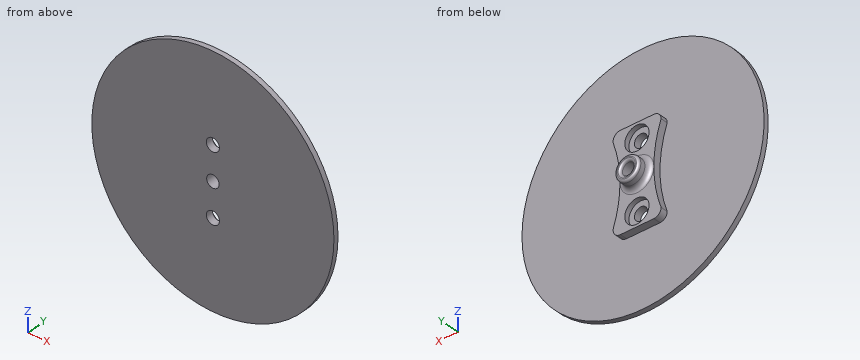
Autodesk Inventor part; units mm, degrees
ref_plane "YZ Plane" through (0, 0, 0) normal (1, 0, 0) x (0, 1, 0)
ref_plane "XZ Plane" through (0, 0, 0) normal (0, 1, 0) x (-1, 0, 0)
ref_plane "XY Plane" through (0, 0, 0) normal (0, 0, 1) x (1, 0, 0)
sketch "Boceto1" plane through (0, 0, 0) normal (0, 1, 0) x (-1, 0, 0)
  circle A0 centre (0, 0) radius 2.7
  line L0 (10, 20) -> (-10, 20)
  line L1 (-10, 20) -> (-10, -20)
  line L2 (-10, -20) -> (10, -20)
  line L3 (10, -20) -> (10, 20)
  line L4 (10, 20) -> (-10, -20) construction
  line L5 (-10, 20) -> (10, -20) construction
  circle A1 centre (0, 14) radius 2.7
  circle A2 centre (0, -14) radius 2.7
  dimension "d0" = 5.4
  dimension "d1" = 20
  dimension "d2" = 40
  dimension "d3" = 6
  dimension "d4" = 6
extrude "Extrusión1" add sketch "Boceto1" along normal blind 5
sketch "Boceto2" plane through (0, 5, 0) normal (0, 1, 0) x (1, 0, 0)
  circle A0 centre (0, 0) radius 2.7
  circle A1 centre (0, 0) radius 2.7
  circle A2 centre (0, 0) radius 5
  dimension "d21" = 2
  dimension "d22" = 0
  dimension "d7" = 10
extrude "Extrusión2" add sketch "Boceto2" along normal blind 5
sketch "Boceto3" plane through (0, 10, 0) normal (0, 1, 0) x (1, 0, 0)
  circle A0 centre (0, 0) radius 2.575
  circle A1 centre (0, 0) radius 2.7
  dimension "d10" = 5.15
extrude "Extrusión3" add sketch "Boceto3" against normal up to surface (10 mm away)
fillet "Empalme1" radius 3 4 edges at (-10, 2.5, -20) (10, 2.5, -20) (10, 2.5, 20) (-10, 2.5, 20)
fillet "Empalme2" radius 2 1 edges at (-5, 5, 0)
sketch "Boceto4" plane through (0, 5, 0) normal (0, 1, 0) x (1, 0, 0)
  line L0 (10, -17) -> (10, 17)
  arc A0 (10, 17) -> (10, -17) centre (56.6667, 0) ccw
  line L1 (10, -17) -> (10, 17)
  line L2 (-10, 17) -> (-10, -17)
  arc A1 (-7, 20) -> (-10, 17) centre (-7, 17) ccw
  arc A2 (-10, -17) -> (-10, 17) centre (-56.6667, 0) ccw
  line L3 (-10, 17) -> (-10, -17)
  point P0 (0, 0)
extrude "Extrusión4" cut sketch "Boceto4" against normal through all
fillet "Empalme3" radius 3 2 edges at (10, 2.5, 17) (10, 2.5, -17)
fillet "Empalme4" radius 1 2 edges at (-5, 10, 0) (-2.575, 10, 0)
sketch "Boceto5" plane through (0, 5, 0) normal (0, 1, 0) x (1, 0, 0)
  circle A0 centre (0, -14) radius 2.7
  circle A1 centre (0, -14) radius 5
  circle A2 centre (0, 14) radius 2.7
  circle A3 centre (0, 14) radius 5
  point P0 (0, 0)
  dimension "d19" = 10
  dimension "d20" = 10
extrude "Extrusión5" cut sketch "Boceto5" against normal blind 2 contours A0 | A1 | A2 | A3
sketch "Boceto7" plane through (0, 0, 0) normal (0, -1, 0) x (1, 0, 0)
  circle A0 centre (0, 0) radius 2.575
  circle A1 centre (0, 0) radius 50
  circle A2 centre (0, -14) radius 2.7
  circle A3 centre (0, 14) radius 2.7
  circle A4 centre (0, 0) radius 2.575
  arc A5 (6.8191, -20) -> (9.6585, -16.0316) centre (6.8191, -17) ccw
  arc A6 (9.6585, 16.0316) -> (9.6585, -16.0316) centre (56.6667, 0) ccw
  arc A7 (9.6585, 16.0316) -> (6.8191, 20) centre (6.8191, 17) ccw
  line L0 (-7, 20) -> (6.8191, 20)
  arc A8 (-7, 20) -> (-10, 17) centre (-7, 17) ccw
  arc A9 (-10, -17) -> (-10, 17) centre (-56.6667, 0) ccw
  arc A10 (-10, -17) -> (-7, -20) centre (-7, -17) ccw
  line L1 (6.8191, -20) -> (-7, -20)
  dimension "d24" = 100
extrude "Extrusión6" add sketch "Boceto7" against normal blind 2 contours A1
properties part number "plataforma"
Source: CAD feature listing. Evaluate the final solid. Frame: model axes, mm. Give positions to 0.01 mm unless a question says otherwise; leave off trailing zeros. Order: outer loops, then holes, each group sorted by start corner. A loop starts at its lowest first (then second) coordinate and runs counter-clockwise, first axis right, second up. Notation, with made-up numbers: (-37, 56) -> (10, 56) arc R30 ccw to (10, 92) -> close; hole circle Ø1 at (1.25, 8.5). An arc over 180 degrees is marked (long way). Write item = value, one per line.
Item 1: Section query B-B (x = 0). State how many separate pieces and enclosed holes the cut face has, then the cut area to 3 significant figures.
Check result:
separate_pieces = 4
enclosed_holes = 0
area = 247 mm²
Item 2: Contact query for flat-ended pins moving along their axis: pin 1 (9 mm diameter, centred on x = 0, z = 14, fed in from +Y); pin 2 (5 mm diameter, centred on x = 12.5, z = 15, fed in from -Y); pin 3 (11 mm diameter, centred on x = -1.5, z = 12, fed in from +Y); pin 4 (2.5 mm diameter, centred on x = -3.5, y = 3, fed in from +Z). Output: stop coordinate, or through.
Check result:
pin_1 = 3
pin_2 = 0
pin_3 = 5.04
pin_4 = 49.92
Item 3: Section query D-D (z = 38). Output: boundary loops of the cut face in (x, y), then the cut area to 3 significant figures.
Check result:
outline = (-32.5, 0) -> (32.5, 0) -> (32.5, 2) -> (-32.5, 2) -> close
area = 130 mm²
Item 4: Section query A-A (z = 14). Output: boundary loops of the cut face in (x, y), then the cut area to 3 significant figures.
Check result:
outline = (-48, 0) -> (-2.7, 0) -> (-2.7, 3) -> (-5, 3) -> (-5, 5) -> (-9.01, 5) -> (-9.01, 2) -> (-48, 2) -> close; (2.7, 0) -> (48, 0) -> (48, 2) -> (9.01, 2) -> (9.01, 5) -> (5, 5) -> (5, 3) -> (2.7, 3) -> close
area = 210 mm²
Item 5: Ray query, probe 1 along Z at (x, y) = (0, 3.75) (3 decimals); probe 2 along Z at (x, y) = (0, 2.4) (3 decimals); probe 3 along X at (y, z) = (3.6, -14). Return the intervals inside material, ascending.
Check result:
probe_1 = -20 to -19, -9 to -2.575, 2.575 to 9, 19 to 20
probe_2 = -20 to -16.7, -11.3 to -2.575, 2.575 to 11.3, 16.7 to 20
probe_3 = -9.01 to -5, 5 to 9.01
Item 6: Section query C-C (x = -33.5). Output: boundary loops of the cut face in (y, z).
Check result:
outline = (0, -37.12) -> (2, -37.12) -> (2, 37.12) -> (0, 37.12) -> close
